Autodesk Inventor part; units mm, degrees
ref_plane "YZ Plane" through (0, 0, 0) normal (1, 0, 0) x (0, 1, 0)
ref_plane "XZ Plane" through (0, 0, 0) normal (0, 1, 0) x (-1, 0, 0)
ref_plane "XY Plane" through (0, 0, 0) normal (0, 0, 1) x (1, 0, 0)
sketch "Sketch1" plane through (0, 0, 0) normal (0, 1, 0) x (-1, 0, 0)
  circle A0 centre (0, 0) radius 3
  dimension "d0" = 6
extrude "Extrusion1" add sketch "Sketch1" along normal blind 2
sketch "Sketch2" plane through (0, 0, 0) normal (0, -1, 0) x (1, 0, 0)
  circle A0 centre (0, 0) radius 1.5
  dimension "d3" = 3
extrude "Extrusion2" add sketch "Sketch2" along normal blind 12
chamfer "Chamfer1" distance 0.5 angle 45 1 edges at (-1.5, -12, 0)
fillet "Fillet1" radius 1 1 edges at (3, 2, 0)
properties part number "plastic M3 bolt"
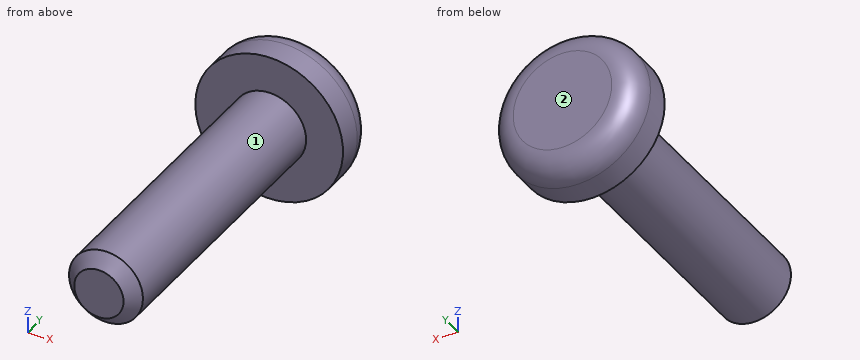
Here's how the part is built. I have some questions about the finished solid (model axes, mm). Face numbers are marked on the shaded views. A direction names the side the tool comes from. Round coordinates to 2 decimals unless told otherwise and drop trailing zeros. Write each loop counter-clockwise with the first axis right and the second up, starting at its lowest first coordinate (ties: lowest second). Pieces come first, ordered by that corner, then holes.
Q1. If we section it at B-B on z = 0: Write out the boundary of the cut face in (x, y).
Q2. If we section it at C-C on y = 0.5: Write out the boundary of the cut face in (x, z), plus the area to 3 significant figures.
Q3. If we section it at D-D on y = -6.25: Write out the boundary of the cut face in (x, z), plus the area to 3 significant figures.
Q4. Which directions (+Z, -Z, +X, -X, +Y, -Y) give clear straight access to the entire face, cutting with the end or side of a thin tool? Please do the marked faces 1 and 2.
Q5. If we section it at A-A on x = 0: Write out the boundary of the cut face in (y, z).
Q6. Will these pins go through, and if not, where does the flat tip stop? P1, Ø2, axis at y = -5.5, z = 0, coming from the -X side; P2, Ø2, axis at y = -2.5, z = 1.5, coming from the +X side; P3, Ø1.5, axis at x = 1.5, y = -1.5, coming from the -Z side.
Q7. Please list where these lines run through material, in increasing order: probe 1 along X at (y, z) = (-11.25, 0.05); probe 2 along Y at (x, z) = (-1.35, -1.05); probe 3 along Z at (x, y) = (-2.2, 1.25).
Answer below:
1. outline: (-3, 0) - (-1.5, 0) - (-1.5, -11.5) - (-1, -12) - (1, -12) - (1.5, -11.5) - (1.5, 0) - (3, 0) - (3, 1) arc R1 ccw to (2, 2) - (-2, 2) arc R1 ccw to (-3, 1) - close
2. outline: circle Ø6 at (0, 0)
2. area: 28.3 mm2
3. outline: circle Ø3 at (0, 0)
3. area: 7.07 mm2
4. face 1: -Y
4. face 2: +Z, -Z, +X, -X, +Y
5. outline: (-12, -1) - (-11.5, -1.5) - (0, -1.5) - (0, -3) - (1, -3) arc R1 ccw to (2, -2) - (2, 2) arc R1 ccw to (1, 3) - (0, 3) - (0, 1.5) - (-11.5, 1.5) - (-12, 1) - close
6. P1: stops at x = -1.5
6. P2: stops at x = 1.41
6. P3: stops at z = -1.3
7. probe 1: x = -1.5 to 1.5
7. probe 2: y = 0 to 2
7. probe 3: z = -1.99 to 1.99
